from build123d import *

# Parameters (mm, degrees)
EXTRUDE_1_DEPTH     = 20
SKETCH_2_R          = 2.5
CUT_EXTRUDE_4_DEPTH = 20
SKETCH_3_W          = 37.700616616
SKETCH_3_H          = 20
EXTRUDE_3_DEPTH     = 1
SKETCH_4_R          = 3
EXTRUDE_4_DEPTH     = 3.5


with BuildPart() as part:
    # 草图1 → 凸台-拉伸1 (new body)
    with BuildSketch(Plane.XY):
        Polygon((20, 0), (-20, 0), (-20, 27.5), (-27.25, 27.5), (-27.25, 30.5), (-20, 30.5), (-20, 40), (20, 40), (20, 30.5), (27.25, 30.5), (27.25, 27.5), (20, 27.5), align=None)
    extrude(amount=-EXTRUDE_1_DEPTH)

    # 草图2 → 切除-拉伸4 (cut)
    with BuildSketch(Plane(origin=(0, 30.5, 0), x_dir=(1, 0, 0), z_dir=(0, 1, 0))):
        with Locations((-24.76, 15)):
            Circle(SKETCH_2_R)
        with Locations((-24.76, 5)):
            Circle(SKETCH_2_R)
        with Locations((24.76, 5)):
            Circle(SKETCH_2_R)
        with Locations((24.76, 15)):
            Circle(SKETCH_2_R)
    extrude(amount=-CUT_EXTRUDE_4_DEPTH, mode=Mode.SUBTRACT)

    # 草图3 → 凸台-拉伸3 (add)
    with BuildSketch(Plane(origin=(0, 40, 0), x_dir=(1, 0, 0), z_dir=(0, 1, 0))):
        with Locations((0.280093734, 10)):
            Rectangle(SKETCH_3_W, SKETCH_3_H)
    extrude(amount=EXTRUDE_3_DEPTH)

    # 草图4 → 凸台-拉伸4 (add)
    with BuildSketch(Plane(origin=(0, 41, 0), x_dir=(1, 0, 0), z_dir=(0, 1, 0))):
        with Locations((11.329785426, 10)):
            Circle(SKETCH_4_R)
    extrude(amount=EXTRUDE_4_DEPTH)


solid = part.part
Geometry: final body of the model. Coordinates: model frame, mm. A direction names the side the tool comes from. Coordinates: 2 decimals unless noted, no trailing zeros. Order: outer loops, then holes, each group sorted by start corner. A loop starts at its lowest first (then second) coordinate and runs counter-clockwise, first axis right, second up.
1) Section A-A (x = 24.76). Return loops of the section in (y, z), then the cut area to 3 significant figures.
Result sheet:
outline: (27.5, -20) - (30.5, -20) - (30.5, -17.5) - (27.5, -17.5) - close; (27.5, -12.5) - (30.5, -12.5) - (30.5, -7.5) - (27.5, -7.5) - close; (27.5, -2.5) - (30.5, -2.5) - (30.5, 0) - (27.5, 0) - close
area: 30.0 mm2
2) Ray query, probe 1 along Z at (x, y) = (24.76, 29); probe 2 along Z at (x, y) = (24, 28); probe 3 along Y at (x, z) = (-17, -5). Return the intervals inside material, ascending.
Result sheet:
probe 1: z = -20 to -17.5, -12.5 to -7.5, -2.5 to 0
probe 2: z = -20 to -17.38, -12.62 to -7.38, -2.62 to 0
probe 3: y = 0 to 41
3) Section D-D (y = 23). Return loops of the section in (x, z), then the cut area to 3 significant figures.
Result sheet:
outline: (-20, -20) - (20, -20) - (20, 0) - (-20, 0) - close
area: 800 mm2
4) Draft query along Z for faces 1 (the flat face through (-24, 30.5, -10)), 2 (the cylindrical face through (22.262, 29.021, -5.107)), 3 (the cylindrical face through (14.1, 42.73, -8.85)). Return one class per face: released by +Z, released by -Z, zero draft, split by the parting line, or undercut.
Result sheet:
face 1: zero draft
face 2: undercut
face 3: split by the parting line
5) Section C-C (z = -4). Return loops of the section in (x, y), then the cut area to 3 significant figures.
Result sheet:
outline: (-27.25, 27.5) - (-27.05, 27.5) - (-27.05, 30.5) - (-27.25, 30.5) - close; (-22.47, 27.5) - (-20, 27.5) - (-20, 0) - (20, 0) - (20, 27.5) - (22.47, 27.5) - (22.47, 30.5) - (20, 30.5) - (20, 40) - (19.13, 40) - (19.13, 41) - (-18.57, 41) - (-18.57, 40) - (-20, 40) - (-20, 30.5) - (-22.47, 30.5) - close; (27.05, 27.5) - (27.25, 27.5) - (27.25, 30.5) - (27.05, 30.5) - close
area: 1,650 mm2
6) Section B-B (z = -10). Return loops of the section in (x, y), then the cut area to 3 significant figures.
Result sheet:
outline: (-27.25, 27.5) - (-20, 27.5) - (-20, 0) - (20, 0) - (20, 27.5) - (27.25, 27.5) - (27.25, 30.5) - (20, 30.5) - (20, 40) - (19.13, 40) - (19.13, 41) - (14.33, 41) - (14.33, 44.5) - (8.33, 44.5) - (8.33, 41) - (-18.57, 41) - (-18.57, 40) - (-20, 40) - (-20, 30.5) - (-27.25, 30.5) - close
area: 1,700 mm2
7) Set-up query: faces 4 (the flat face through (-20, 35, -10)), 5 (the flat face through (24, 27.5, -10)), 6 (the flat face through (20, 35, -10)). Return all of +Z, -Z, +X, -X, +Y, -Y with unobstructed straight access to the full face (end or side cutting, diameter ignored); none if empty.
Result sheet:
face 4: +Z, -Z, -X, +Y
face 5: +Z, -Z, +X, -Y
face 6: +Z, -Z, +X, +Y
8) First-contact query: P1, Ø4, axis at x = 0, y = 31.5, coming from the +Z side; P2, Ø5, axis at y = 36, z = -7.5, coming from the -X side; P3, Ø6, axis at x = 24.76, z = -15, coming from the -Y side; P4, Ø8, axis at x = 24.5, z = -8.5, coming from the +Y side. Flat tips, straight axial feed; report the tip coordinate or a pass-through.
Result sheet:
P1: stops at z = 0
P2: stops at x = -20
P3: stops at y = 27.5
P4: stops at y = 30.5
